For this review, take the finished solid that the model builds, in its own axes (mm). Round coordinates to 2 decimals unless told otherwise and drop trailing zeros. Loops run counter-clockwise (first coordinate to the right, second up) from the corner with the lowest first, then second, coordinate; pieces in that order, holes last.
```python
from build123d import *

# Parameters (mm, degrees)
SALIENTE_EXTRUIR1_DEPTH = 3


with BuildPart() as part:
    # Croquis1 → Saliente-Extruir1 (new body)
    with BuildSketch(Plane(origin=(0, 0, 0), x_dir=(1, 0, 0), z_dir=(0, 1, 0))):
        with BuildLine():
            Line((0, 33), (-5.331406318, 33))
            ThreePointArc((-5.331406318, 33), (-12.593971099, 31.555386046), (-18.750876228, 27.441473563))
            Line((-18.750876228, 27.441473563), (-64.799895827, -18.607546035))
            ThreePointArc((-64.799895827, -18.607546035), (-69.135552051, -23.128851505), (-73.277942785, -27.827863853))
            ThreePointArc((-73.277942785, -27.827863853), (-74.646122538, -30.183582463), (-75.121480816, -32.86599938))
            Line((-75.121480816, -32.86599938), (-75.121480816, -51.309071299))
            ThreePointArc((-75.121480816, -51.309071299), (-74.581521028, -52.612649541), (-73.277942785, -53.152609329))
            Line((-73.277942785, -53.152609329), (-67.7929112, -53.152609329))
            ThreePointArc((-67.7929112, -53.152609329), (-67.328497374, -53.097942153), (-66.88947174, -52.936929127))
            Line((-66.88947174, -52.936929127), (-6.151808223, -22.184144776))
            ThreePointArc((-6.151808223, -22.184144776), (-5.489025915, -21.643589172), (-5.112658875, -20.875586177))
            Line((-5.112658875, -20.875586177), (0, 0))
            Line((0, 0), (38.425, 0))
            Line((38.425, 0), (38.425, 115))
            Line((38.425, 115), (41.425, 115))
            Line((41.425, 115), (41.425, 0))
            Line((41.425, 0), (60, 0))
            Line((60, 0), (60, 210))
            Line((60, 210), (59.5, 210))
            Line((59.5, 210), (59.5, 213))
            Line((59.5, 213), (59, 213))
            Line((59, 213), (59, 216))
            Line((59, 216), (58.5, 216))
            Line((58.5, 216), (58.5, 219))
            Line((58.5, 219), (58, 219))
            Line((58, 219), (58, 222))
            Line((58, 222), (57.5, 222))
            Line((57.5, 222), (57.5, 225))
            Line((57.5, 225), (57, 225))
            Line((57, 225), (57, 228))
            Line((57, 228), (56.5, 228))
            Line((56.5, 228), (56.5, 231))
            Line((56.5, 231), (56, 231))
            Line((56, 231), (56, 234))
            Line((56, 234), (55.5, 234))
            Line((55.5, 234), (55.5, 237))
            Line((55.5, 237), (55, 237))
            Line((55, 237), (55, 240))
            Line((55, 240), (54.5, 240))
            Line((54.5, 240), (54.5, 243))
            Line((54.5, 243), (54, 243))
            Line((54, 243), (54, 246))
            Line((54, 246), (53.5, 246))
            Line((53.5, 246), (53.5, 249))
            Line((53.5, 249), (53, 249))
            Line((53, 249), (53, 252))
            Line((53, 252), (52.5, 252))
            Line((52.5, 252), (52.5, 255))
            Line((52.5, 255), (52, 255))
            Line((52, 255), (52, 258))
            Line((52, 258), (51.5, 258))
            Line((51.5, 258), (51.5, 261))
            Line((51.5, 261), (51, 261))
            Line((51, 261), (51, 264))
            Line((51, 264), (50.5, 264))
            Line((50.5, 264), (50.5, 267))
            ThreePointArc((50.5, 267), (39.925, 277.575), (29.35, 267))
            Line((29.35, 267), (29.35, 264))
            Line((29.35, 264), (28.27, 264))
            Line((28.27, 264), (28.27, 261))
            Line((28.27, 261), (26.35, 261))
            Line((26.35, 261), (26.35, 258))
            Line((26.35, 258), (24.78, 258))
            Line((24.78, 258), (24.78, 255))
            Line((24.78, 255), (23.58, 255))
            Line((23.58, 255), (23.58, 252))
            Line((23.58, 252), (22.19, 252))
            Line((22.19, 252), (22.19, 249))
            Line((22.19, 249), (20.92, 249))
            Line((20.92, 249), (20.92, 246))
            Line((20.92, 246), (19.9, 246))
            Line((19.9, 246), (19.9, 243))
            Line((19.9, 243), (18.75, 243))
            Line((18.75, 243), (18.75, 240))
            Line((18.75, 240), (17.37, 240))
            Line((17.37, 240), (17.37, 237))
            Line((17.37, 237), (16.1, 237))
            Line((16.1, 237), (16.1, 234))
            Line((16.1, 234), (14.35, 234))
            Line((14.35, 234), (14.35, 231))
            Line((14.35, 231), (12.73, 231))
            Line((12.73, 231), (12.73, 228))
            Line((12.73, 228), (9.53, 228))
            Line((9.53, 228), (9.53, 225))
            Line((9.53, 225), (6.82, 225))
            Line((6.82, 225), (6.82, 222))
            Line((6.82, 222), (4.53, 222))
            Line((4.53, 222), (4.53, 219))
            Line((4.53, 219), (3.37, 219))
            Line((3.37, 219), (3.37, 216))
            Line((3.37, 216), (2.09, 216))
            Line((2.09, 216), (2.09, 213))
            Line((2.09, 213), (1.36, 213))
            Line((1.36, 213), (1.36, 210))
            Line((1.36, 210), (0, 210))
            Line((0, 210), (0, 33))
        make_face()
    extrude(amount=SALIENTE_EXTRUIR1_DEPTH)


solid = part.part
```
(1) For L1, parallel to X at y = 0.4, z = -44.5 (3 decimals); L2, parallel to X at y = 1.55, z = -233.5; L3, parallel to X at y = 0.5, z = -5 (3 decimals), list the stretches that pass through material, from the lowest coordinate up.
(2) Add section A-A (z = -15). Give the boundary of the cut face in (x, y) (3 decimals).
(3) Add section B-B (z = -155). Give the boundary of the cut face in (x, y), plus the area to 3 significant figures.
(4) Insertion check: pin 1 Ø1.3 at (x, y) = (24, 1) entering from -Z; pin 2 Ø0.7 at (x, y) = (18, 1.5) entering from -Z; pin 3 Ø0.9 at (y, z) = (2, -232.5) entering from +X. Each pin has a flat end and moves straight along its axis. Give the tip position at first contact, or say it passes through.
(5) Add section C-C (x = 47.5). Give the boundary of the cut face in (y, z), plus the area to 3 significant figures.
Outcome:
1. L1: x = 0 to 38.425, 41.425 to 60
1. L2: x = 14.35 to 56
1. L3: x = -41.192 to 38.425, 41.425 to 60
2. outline: (-31.192, 0) - (38.425, 0) - (38.425, 3) - (-31.192, 3) - close; (41.425, 0) - (60, 0) - (60, 3) - (41.425, 3) - close
3. outline: (0, 0) - (60, 0) - (60, 3) - (0, 3) - close
3. area: 180 mm2
4. pin 1: stops at z = -255
4. pin 2: stops at z = -240
4. pin 3: stops at x = 56
5. outline: (0, -274.38) - (3, -274.38) - (3, 0) - (0, 0) - close
5. area: 823 mm2
